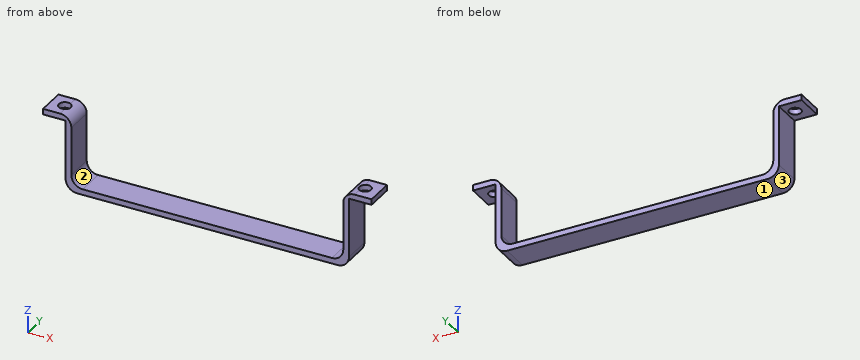
from build123d import *

# Parameters (mm, degrees)
F1_DEPTH    = 12.7
F2_R        = 2.667
F3_R        = 2.667
F4_DEPTH    = 25.4
F5_T1_DEPTH = 12.7
F5_T3_DEPTH = 38.1


# Not quite as in the source:
# - a fillet or chamfer that OpenCascade refuses, or shapes differently, is made with other operations: its cross-section is extruded or revolved along the edge and cut away or added


with BuildPart() as f1:
    # F0 (on Front) → F1 (new body)
    with BuildSketch(Plane.XZ):
        Polygon((121.92, 0), (0, 0), (0, 31.75), (-12.7, 31.75), (-12.7, 29.2099993676), (-2.5400006324, 29.2099993676), (-2.5400006324, -2.5400006324), (124.4600006324, -2.5400006324), (124.4600006324, 29.2099993676), (134.62, 29.2099993676), (134.62, 31.75), (121.92, 31.75), align=None)
    extrude(amount=F1_DEPTH)

    # F2 (on face) + F3 (on face) → F4 (cut)
    with BuildSketch(Plane.XY.offset(31.75)):
        with Locations((-6.35, -6.35)):
            Circle(F2_R)
    with BuildSketch(Plane.XY.offset(31.75)):
        with Locations((128.27, -6.35)):
            Circle(F3_R)
    extrude(amount=-F4_DEPTH, mode=Mode.SUBTRACT)

    # F5: fillet of radius 5.08 on 6 edges, made by hand

    # F5_s2 → F5_t1 (join)
    with BuildSketch(Plane.XZ):
        with BuildLine():
            ThreePointArc((5.08, 0), (1.4878975516, 1.4878975516), (0, 5.08))
            Line((0, 5.08), (0, 0))
            Line((0, 0), (5.08, 0))
        make_face()
        with BuildLine():
            ThreePointArc((116.84, 0), (120.4321024484, 1.4878975516), (121.92, 5.08))
            Line((121.92, 5.08), (121.92, 0))
            Line((121.92, 0), (116.84, 0))
        make_face()
    extrude(amount=F5_T1_DEPTH)

    # F5_s4 → F5_t3 (cut)
    with BuildSketch(Plane.XZ.offset(-12.7)):
        with BuildLine():
            ThreePointArc((-2.5400006324, 2.5399993676), (-1.0521030808, -1.0521030808), (2.5399993676, -2.5400006324))
            Line((2.5399993676, -2.5400006324), (-2.5400006324, -2.5400006324))
            Line((-2.5400006324, -2.5400006324), (-2.5400006324, 2.5399993676))
        make_face()
        with BuildLine():
            ThreePointArc((119.3800006324, -2.5400006324), (122.9721030808, -1.0521030808), (124.4600006324, 2.5399993676))
            Line((124.4600006324, 2.5399993676), (124.4600006324, -2.5400006324))
            Line((124.4600006324, -2.5400006324), (119.3800006324, -2.5400006324))
        make_face()
        with BuildLine():
            ThreePointArc((127, 31.75), (123.4078975516, 30.2621024484), (121.92, 26.67))
            Line((121.92, 26.67), (121.92, 31.75))
            Line((121.92, 31.75), (127, 31.75))
        make_face()
        with BuildLine():
            ThreePointArc((0, 26.67), (-1.4878975516, 30.2621024484), (-5.08, 31.75))
            Line((-5.08, 31.75), (0, 31.75))
            Line((0, 31.75), (0, 26.67))
        make_face()
    extrude(amount=F5_T3_DEPTH, mode=Mode.SUBTRACT)


solid = f1.part
Model file for the job. Use its own axes, mm. Face numbers are marked on the shaded views. Give positions to 0.01 mm unless a question says otherwise; leave off trailing zeros. Order: outer loops, then holes, each group sorted by start corner. A loop starts at its lowest first (then second) coordinate and runs counter-clockwise, first axis right, second up. Notation, with made-up numbers: (4.25, 42.5) - (20.25, 42.5) arc R5 ccw to (20.25, 47.5) - close; hole circle Ø6 at (10.5, -20). An arc over 180 degrees is marked (long way). Write item = value, one per line. Start each with the question number.
1. Cut at B-B, the plane z = 18. List the corners of the cut face in (x, y).
2. Cut at A-A, the plane x = -6.35. List the corners of the cut face in (y, z).
3. Probe line 1 along X through (y, z) = (-11.25, 11); line 2 along Y through (x, z) = (-6.35, 30.5); line 3 along X through (y, z) = (-6.35, 30.7). List the from-to ranges inside material, lowest first.
4. Drop flat-ended pins along their axis: P1, Ø6.5, axis at x = 44.5, y = -7, coming from the +Z side; P2, Ø3, axis at x = -9, y = -8.5, coming from the -Z side; P3, Ø1.5, axis at y = -9, z = 14, coming from the -X side. Give the stop position or say it passes through.
5. Cut at C-C, the plane y = -6.35. List the corners of the cut face in (x, z), and give its area (3 significant figures).
6. Cut at D-D, the plane x = 70.5. List the corners of the cut face in (y, z).
7. Two-plate mould, pull along X, no slides. Class the marked faces 1, 2 and 3: pulls with the +X half, pulls with the -X half, needs draft (parallel to the pull), parting line crosses it, or undercut.
Taken from the geometry:
q1.outline = (-2.54, -12.7) - (0, -12.7) - (0, 0) - (-2.54, 0) - close; (121.92, -12.7) - (124.46, -12.7) - (124.46, 0) - (121.92, 0) - close
q2.outline = (-12.7, 29.21) - (-9.02, 29.21) - (-9.02, 31.75) - (-12.7, 31.75) - close; (-3.68, 29.21) - (0, 29.21) - (0, 31.75) - (-3.68, 31.75) - close
q3.line_1 = -2.54 to 0, 121.92 to 124.46
q3.line_2 = -12.7 to -9.02, -3.68 to 0
q3.line_3 = -12.7 to -9.02, -3.68 to -1.99, 123.91 to 125.6, 130.94 to 134.62
q4.P1 = 0
q4.P2 = 29.21
q4.P3 = -2.54
q5.outline = (-12.7, 29.21) - (-9.02, 29.21) - (-9.02, 31.75) - (-12.7, 31.75) - close; (-3.68, 29.21) - (-2.54, 29.21) - (-2.54, 2.54) arc R5.08 ccw to (2.54, -2.54) - (119.38, -2.54) arc R5.08 ccw to (124.46, 2.54) - (124.46, 29.21) - (125.6, 29.21) - (125.6, 31.55) arc R5.08 ccw to (121.92, 26.67) - (121.92, 5.08) arc R5.08 cw to (116.84, 0) - (5.08, 0) arc R5.08 cw to (0, 5.08) - (0, 26.67) arc R5.08 ccw to (-3.68, 31.55) - close; (130.94, 29.21) - (134.62, 29.21) - (134.62, 31.75) - (130.94, 31.75) - close
q5.area = 497 mm²
q6.outline = (-12.7, -2.54) - (0, -2.54) - (0, 0) - (-12.7, 0) - close
q7.face_1 = needs draft
q7.face_2 = undercut
q7.face_3 = pulls with the -X half
